Geometry: final body of the model. Coordinates: model frame, mm. Face numbers are marked on the shaded views. A direction names the side the tool comes from. Coordinates: 2 decimals unless noted, no trailing zeros. Loops run counter-clockwise (first coordinate to the right, second up) from the corner with the lowest first, then second, coordinate; pieces in that order, holes last. Notation, with made-up numbers: (77, -30) - (90, -30) arc R34 cw to (90, 4) - close; hole circle Ø11 at (35, -29). An arc over 180 degrees is marked (long way). Put each result on its own line as item: value. Start each with the question number.
1) Section A-A on y = 11.25. Output: boundary loops of the cut face in (x, z), and give its area (3 significant figures).
2) Section D-D on x = -7. Output: boundary loops of the cut face in (y, z) (3 decimals), and give its area (3 significant figures).
3) Draft query along Z for the marked faces 4, 5 and 6. Return one class per face: +Z half, -Z half, draft (parallel to the pull), parting line (faces both ways), or undercut.
4) Section B-B on x = 0. Output: boundary loops of the cut face in (y, z) (3 decimals), and give its area (3 significant figures).
5) Contact query for flat-ended pins moving along their axis: pin 1 Ø5 at (x, y) = (8, 10.5) entering from -Z; pin 2 Ø4 at (y, z) = (15.5, -2) entering from -X; pin 3 Ø5 at (x, y) = (-7, 13.5) entering from -Z. Output: stop coordinate, or through.
6) Section C-C on z = -7.5. Output: boundary loops of the cut face in (x, y) (3 decimals), and give its area (3 significant figures).
7) Material intervals for line 1 along Z through (x, y) = (-1.5, 13.75); line 2 along X through (y, z) = (5.5, 4.5); line 3 along Z through (x, y) = (-2.75, 14.5), sorted ascending. Write a range as from..to.
8) Reachability of the marked faces 1, 2 and 3 from +Z, -Z, +X, -X, +Y, -Y: full face, straight path, thin tool, end or side. Return the list, or none.
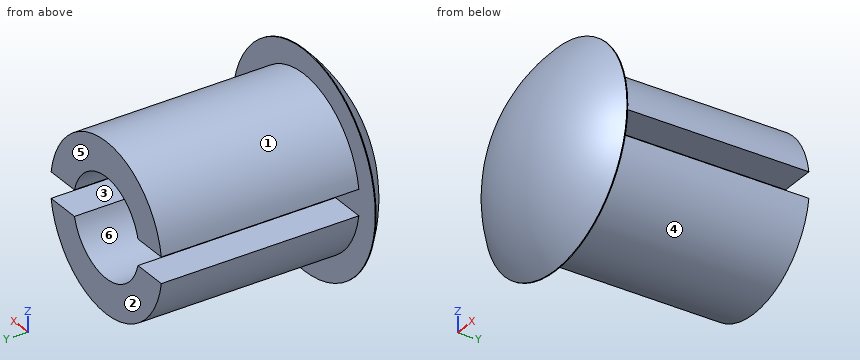
```python
from build123d import *

# Parameters (mm, degrees)
SKETCH1_R           = 12.5
BOSS_EXTRUDE1_DEPTH = 0.1
DOME1_FACE_RADIUS   = 12.5
DOME1_HEIGHT        = 5
SKETCH2_R           = 9.75
BOSS_EXTRUDE2_DEPTH = 23
CUT_EXTRUDE1_REACH  = 35.198
SKETCH3_W           = 22.394577403
SKETCH3_H           = 3


# Read off the part's stored shape, not the designer's step: Shell3
with BuildPart() as part:
    # Sketch1 → Boss-Extrude1 (new body)
    with BuildSketch(Plane(origin=(0, 0, 0), x_dir=(1, 0, 0), z_dir=(0, 1, 0))):
        with Locations(Location((0, 0, 0), (0, 0, 270))):
            Circle(SKETCH1_R)
    extrude(amount=BOSS_EXTRUDE1_DEPTH)

    # Dome1: a dome of height H over a round flat face of radius A is a cap of a sphere of radius (A * A + H * H) / (2 * H)
    dome1_r = (DOME1_FACE_RADIUS * DOME1_FACE_RADIUS + DOME1_HEIGHT * DOME1_HEIGHT) / (2 * DOME1_HEIGHT)
    dome1_base = Plane((0, 0, 0), z_dir=(0, -1, 0))
    with Locations(dome1_base.offset(DOME1_HEIGHT - dome1_r)):
        dome1_ball = Sphere(dome1_r, mode=Mode.PRIVATE)
    add(split(dome1_ball, bisect_by=dome1_base, keep=Keep.TOP, mode=Mode.PRIVATE))

    # Sketch2 → Boss-Extrude2 (add)
    with BuildSketch(Plane(origin=(0, 0.1, 0), x_dir=(1, 0, 0), z_dir=(0, 1, 0))):
        with Locations(Location((0, 0, 0), (0, 0, 270))):
            Circle(SKETCH2_R)
    extrude(amount=BOSS_EXTRUDE2_DEPTH)

    # Shell3 outline → Shell3 (revolve, cut)
    with BuildSketch(Plane.XY):
        with BuildLine():
            Line((0, 23.1), (0, -1))
            ThreePointArc((0, -1), (2.939346569, -0.690783248), (5.750000013, 0.223328602))
            Line((5.750000013, 0.223328602), (5.75, 23.1))
            Line((5.75, 23.1), (0, 23.1))
        make_face()
    revolve(axis=Axis((0, 0, 0), (0, 1, 0)), mode=Mode.SUBTRACT)

    # Cut-Extrude1: up to this face of the body (flat: up to its plane)
    cut_extrude1_end = Plane(part.part.faces().sort_by_distance((0, 0.1, -12.146446609))[0])
    # Sketch3 → Cut-Extrude1 (cut, up to the picked face)
    with BuildSketch(Plane(origin=(0, 23.1, 0), x_dir=(1, 0, 0), z_dir=(0, 1, 0)), mode=Mode.PRIVATE) as cut_extrude1_sk1:
        with Locations((0.557168459, 0)):
            Rectangle(SKETCH3_W, SKETCH3_H)
    cut_extrude1_tool1 = split(extrude(cut_extrude1_sk1.sketch, amount=-CUT_EXTRUDE1_REACH, mode=Mode.PRIVATE), bisect_by=cut_extrude1_end, keep=Keep.BOTH, mode=Mode.PRIVATE)
    add(cut_extrude1_tool1.solids().sort_by(Axis((0.557168, 23.1, 0), (0, -1, 0)))[0], mode=Mode.SUBTRACT)


solid = part.part
```
Answer block:
1. outline: (-9.63, -1.5) arc R9.75 ccw to (9.63, -1.5) - (5.55, -1.5) arc R5.75 cw to (-5.55, -1.5) - close; (-9.63, 1.5) - (-5.55, 1.5) arc R5.75 cw to (5.55, 1.5) - (9.63, 1.5) arc R9.75 ccw to start
1. area: 171 mm²
2. outline: (0, -10.356) - (0.1, -10.356) - (0.1, -6.787) - (23.1, -6.787) - (23.1, -1.5) - (0.1, -1.5) - (0.1, 1.5) - (23.1, 1.5) - (23.1, 6.787) - (0.1, 6.787) - (0.1, 10.356) - (0, 10.356) arc R16.719 ccw to start
2. area: 296 mm²
3. face 4: -Z half
3. face 5: draft
3. face 6: undercut
4. outline: (0, -12.5) - (0.1, -12.5) - (0.1, -9.75) - (23.1, -9.75) - (23.1, -5.75) - (0.223, -5.75) arc R14.125 cw to (0.223, 5.75) - (23.1, 5.75) - (23.1, 9.75) - (0.1, 9.75) - (0.1, 12.5) - (0, 12.5) arc R18.125 ccw to start
4. area: 264 mm²
5. pin 1: stops at z = -8.05
5. pin 2: stops at x = -9.63
5. pin 3: stops at z = -8.65
6. outline: (-10, 0) arc R16.5 ccw to (10, 0) - (10, 0.1) - (6.23, 0.1) - (6.23, 23.1) - (-6.23, 23.1) - (-6.23, 0.1) - (-10, 0.1) - close
6. area: 335 mm²
7. line 1: z = -9.63..-5.55, 5.55..9.63
7. line 2: x = -8.65..-3.58, 3.58..8.65
7. line 3: z = -9.35..-5.05, 5.05..9.35
8. face 1: +Z, +Y
8. face 2: +Z, -Z, +X, -X, +Y
8. face 3: +X, -X, +Y
